```python
from build123d import *

# Parameters (mm, degrees)
SKETCH_1_W          = 45
SKETCH_1_H          = 10
EXTRUDE_1_DEPTH     = 5
SKETCH_2_W          = 5
SKETCH_2_H          = 4
EXTRUDE_2_DEPTH     = 11
SKETCH_3_W          = 5
SKETCH_3_H          = 2
CUT_EXTRUDE_1_DEPTH = 3
SKETCH_4_W          = 5
SKETCH_4_H          = 2
CUT_EXTRUDE_2_DEPTH = 3
SKETCH_5_R          = 1.25
CUT_EXTRUDE_3_DEPTH = 10
SKETCH_6_R          = 1.65
CUT_EXTRUDE_4_DEPTH = 5
SKETCH_7_W          = 5
SKETCH_7_H          = 4
EXTRUDE_3_DEPTH     = 11
SKETCH_8_W          = 5
SKETCH_8_H          = 2
CUT_EXTRUDE_5_DEPTH = 3
SKETCH_9_W          = 5
SKETCH_9_H          = 2
CUT_EXTRUDE_6_DEPTH = 3
CUT_EXTRUDE_START   = -5
SKETCH_11_R         = 1.25
CUT_EXTRUDE_7_DEPTH = 5


with BuildPart() as part:
    # Эскиз1 → Бобышка-Вытянуть1 (new body)
    with BuildSketch(Plane.XY):
        Rectangle(SKETCH_1_W, SKETCH_1_H)
    extrude(amount=EXTRUDE_1_DEPTH)

    # Эскиз2 → Бобышка-Вытянуть2 (add)
    with BuildSketch(Plane.XY.offset(5)):
        with Locations((-10, 3)):
            Rectangle(SKETCH_2_W, SKETCH_2_H)
        with Locations((10, 3)):
            Rectangle(SKETCH_2_W, SKETCH_2_H)
    extrude(amount=EXTRUDE_2_DEPTH)

    # Эскиз3 → Вырез-Вытянуть1 (cut)
    with BuildSketch(Plane.XY.offset(16)):
        with Locations((-10, 2)):
            Rectangle(SKETCH_3_W, SKETCH_3_H)
    extrude(amount=-CUT_EXTRUDE_1_DEPTH, mode=Mode.SUBTRACT)

    # Эскиз4 → Вырез-Вытянуть2 (cut)
    with BuildSketch(Plane.XY.offset(16)):
        with Locations((10, 2)):
            Rectangle(SKETCH_4_W, SKETCH_4_H)
    extrude(amount=-CUT_EXTRUDE_2_DEPTH, mode=Mode.SUBTRACT)

    # Эскиз5 → Вырез-Вытянуть3 (cut)
    with BuildSketch(Plane(origin=(0, 5, 0), x_dir=(1, 0, 0), z_dir=(0, 1, 0))):
        with Locations(Location((-10, -10.5, 0), (0, 0, 270))):
            Circle(SKETCH_5_R)
        with Locations(Location((10, -10.5, 0), (0, 0, 270))):
            Circle(SKETCH_5_R)
    extrude(amount=-CUT_EXTRUDE_3_DEPTH, mode=Mode.SUBTRACT)

    # Эскиз6 → Вырез-Вытянуть4 (cut)
    with BuildSketch(Plane.XY.offset(5)):
        with Locations((-17.5, 0)):
            Circle(SKETCH_6_R)
        with Locations((17.5, 0)):
            Circle(SKETCH_6_R)
    extrude(amount=-CUT_EXTRUDE_4_DEPTH, mode=Mode.SUBTRACT)

    # Эскиз7 → Бобышка-Вытянуть3 (add)
    with BuildSketch(Plane.XY.offset(5)):
        with Locations((-10, -3)):
            Rectangle(SKETCH_7_W, SKETCH_7_H)
        with Locations((10, -3)):
            Rectangle(SKETCH_7_W, SKETCH_7_H)
    extrude(amount=EXTRUDE_3_DEPTH)

    # Эскиз8 → Вырез-Вытянуть5 (cut)
    with BuildSketch(Plane.XY.offset(16)):
        with Locations((-10, -2)):
            Rectangle(SKETCH_8_W, SKETCH_8_H)
    extrude(amount=-CUT_EXTRUDE_5_DEPTH, mode=Mode.SUBTRACT)

    # Эскиз9 → Вырез-Вытянуть6 (cut)
    with BuildSketch(Plane.XY.offset(16)):
        with Locations((10, -2)):
            Rectangle(SKETCH_9_W, SKETCH_9_H)
    extrude(amount=-CUT_EXTRUDE_6_DEPTH, mode=Mode.SUBTRACT)

    # Эскиз11 → Вырез-Вытянуть7 (cut)
    with BuildSketch(Plane.XZ.offset(5).offset(CUT_EXTRUDE_START)):
        with Locations(Location((-10, 10.5, 0), (0, 0, 90))):
            Circle(SKETCH_11_R)
        with Locations(Location((10, 10.5, 0), (0, 0, 90))):
            Circle(SKETCH_11_R)
    extrude(amount=CUT_EXTRUDE_7_DEPTH, mode=Mode.SUBTRACT)


solid = part.part
```
Check sheet for the modelled part. Datum: model origin and axes. Units: mm. A direction names the side the tool comes from. Give positions to 0.01 mm unless a question says otherwise; leave off trailing zeros. Write each loop counter-clockwise with the first axis right and the second up, starting at its lowest first coordinate (ties: lowest second). Pieces come first, ordered by that corner, then holes.
Item 1: Cross-section at C-C (x = 17.5). Enter the section's corners in (y, z), and give its area (3 significant figures).
Item 2: Gauge pin test, flat ends, axial feed: pin 1 (2 mm diameter, centred on y = 3, z = 12.5, fed in from +X); pin 2 (4 mm diameter, centred on x = -15.5, y = -1.5, fed in from +Z); pin 3 (2 mm diameter, centred on y = -2, z = 9.5, fed in from -X). Record the tip position at first contact, or that the pin passes through.
Item 3: Access from +Z, -Z, +X, -X, +Y, -Y to the whole of each face (thin tool, end or side, straight path). Record for faces 5 (the face through (0, -5, 4)), 6 (the face through (10, 2, 13)), 7 (the face through (12.5, 3, 10)), 8 (the face through (7.5, -3, 10)).
Item 4: Cross-section at A-A (x = -10). Enter the section's corners in (y, z), and give its area (3 significant figures).
Item 5: Draft check along X on faces 1 (the face through (12.5, -3, 10)), 2 (the face through (-10, 4, 16)), 3 (the face through (-12.5, -3, 10)), 4 (the face through (0, 0, 5)). Enter one of: released by +X, released by -X, zero draft, split by the parting line, or undercut.
Item 6: Cross-section at B-B (y = -2.5). Enter the section's corners in (x, z).
Item 7: Cross-section at D-D (z = 6). Enter the section's corners in (x, y), and give its area (3 significant figures).
Item 8: Scan lines: L1, parallel to X at y = -2.15, z = 10.5; L2, parallel to X at y = 1.75, z = 7.25; L3, parallel to X at y = -1.5, z = 4.5. Record each from-to range of solid material in increasing order.
Report:
1. outline: (-5, 0) - (-1.65, 0) - (-1.65, 5) - (-5, 5) - close; (1.65, 0) - (5, 0) - (5, 5) - (1.65, 5) - close
1. area: 33.5 mm2
2. pin 1: stops at x = 12.5
2. pin 2: stops at z = 5
2. pin 3: stops at x = -12.5
3. face 5: +Z, -Z, +X, -X, -Y
3. face 6: +Z, +X, -X
3. face 7: +Z, +X, +Y, -Y
3. face 8: +Z, +Y, -Y
4. outline: (-5, 0) - (5, 0) - (5, 9.25) - (1, 9.25) - (1, 5) - (-1, 5) - (-1, 9.25) - (-5, 9.25) - close; (-5, 11.75) - (-1, 11.75) - (-1, 13) - (-3, 13) - (-3, 16) - (-5, 16) - close; (1, 11.75) - (5, 11.75) - (5, 16) - (3, 16) - (3, 13) - (1, 13) - close
4. area: 106 mm2
5. face 1: released by +X
5. face 2: zero draft
5. face 3: released by -X
5. face 4: undercut
6. outline: (-22.5, 0) - (22.5, 0) - (22.5, 5) - (12.5, 5) - (12.5, 13) - (7.5, 13) - (7.5, 5) - (-7.5, 5) - (-7.5, 13) - (-12.5, 13) - (-12.5, 5) - (-22.5, 5) - close; hole circle Ø2.5 at (-10, 10.5); hole circle Ø2.5 at (10, 10.5)
7. outline: (-12.5, -5) - (-7.5, -5) - (-7.5, -1) - (-12.5, -1) - close; (-12.5, 1) - (-7.5, 1) - (-7.5, 5) - (-12.5, 5) - close; (7.5, -5) - (12.5, -5) - (12.5, -1) - (7.5, -1) - close; (7.5, 1) - (12.5, 1) - (12.5, 5) - (7.5, 5) - close
7. area: 80.0 mm2
8. L1: x = -12.5 to -11.25, -8.75 to -7.5, 7.5 to 8.75, 11.25 to 12.5
8. L2: x = -12.5 to -7.5, 7.5 to 12.5
8. L3: x = -22.5 to -18.19, -16.81 to 16.81, 18.19 to 22.5
